```python
from build123d import *

# Parameters (mm, degrees)
BOSS_EXTRUDE1_DEPTH = 25.4
BOSS_EXTRUDE2_DEPTH = 12.7


with BuildPart() as part:
    # Sketch1 → Boss-Extrude1 (new body)
    with BuildSketch(Plane.XY):
        with BuildLine():
            Line((-4.826, 0.016704998), (-4.826, -3.044495583))
            ThreePointArc((-4.826, -3.044495583), (0, -5.698295002), (4.826, -3.044495583))
            Line((4.826, -3.044495583), (4.826, 0.016704998))
            Line((4.826, 0.016704998), (4.826, 3.07790558))
            ThreePointArc((4.826, 3.07790558), (0, 5.731704998), (-4.826, 3.07790558))
            Line((-4.826, 3.07790558), (-4.826, 0.016704998))
        make_face()
    extrude(amount=BOSS_EXTRUDE1_DEPTH)

    # Sketch2 → Boss-Extrude2 (add)
    with BuildSketch(Plane.XY.offset(25.4)):
        with BuildLine():
            Line((0.79375, 0), (0.79375, 1.374815329))
            ThreePointArc((0.79375, 1.374815329), (-1.5875, 0), (0.79375, -1.374815329))
            Line((0.79375, -1.374815329), (0.79375, 0))
        make_face()
    extrude(amount=BOSS_EXTRUDE2_DEPTH)


solid = part.part
```
CAD build for the part. Positions are in the model's coordinates, mm. A direction names the side the tool comes from. Coordinates: 2 decimals unless noted, no trailing zeros. Write each loop counter-clockwise with the first axis right and the second up, starting at its lowest first coordinate (ties: lowest second). Pieces come first, ordered by that corner, then holes.
(1) Cut at D-D, the plane y = 2. List the corners of the cut face in (x, z).
(2) Cut at B-B, the plane y = 0. List the corners of the cut face in (x, z).
(3) Cut at A-A, the plane x = 0. List the corners of the cut face in (y, z).
(4) Flat gauge pins, fed straight in: pin 1 (2 mm diameter, centred on y = 0, z = 30, fed in from +X); pin 2 (1 mm diameter, centred on x = 2, z = 9.5, fed in from -Y); pin 3 (3 mm diameter, centred on x = -2.5, z = 7, fed in from +Y). Where does each tip first touch, or does it go through?
(5) Drill centre lines: probe 1 along Z at (x, y) = (1.5, 2.25); probe 2 along Y at (x, z) = (-0.25, 28); probe 3 along Y at (x, z) = (-1.75, 12.5). Where is each one in solid material? Low to high.
(6) Cut at C-C, the plane z = 20.5. List the corners of the cut face in (x, y) (1 decimal), and give its area (3 significant figures).
(7) 3-axis set-ups, long thin cutter, end or side, ignore diameter. For faces 1 (the face through (-1.587, 0.047, 31.661)), 2 (the face through (0.794, 0, 32)), 3 (the face through (4.826, 0, 13)): which of +Z, -Z, +X, -X, +Y, -Y reach the whole face in a straight line?
Geometry says:
1. outline: (-4.83, 0) - (4.83, 0) - (4.83, 25.4) - (-4.83, 25.4) - close
2. outline: (-4.83, 0) - (4.83, 0) - (4.83, 25.4) - (0.79, 25.4) - (0.79, 38.1) - (-1.59, 38.1) - (-1.59, 25.4) - (-4.83, 25.4) - close
3. outline: (-5.7, 0) - (5.73, 0) - (5.73, 25.4) - (1.59, 25.4) - (1.59, 38.1) - (-1.59, 38.1) - (-1.59, 25.4) - (-5.7, 25.4) - close
4. pin 1: stops at x = 0.79
4. pin 2: stops at y = -5.5
4. pin 3: stops at y = 5.64
5. probe 1: z = 0 to 25.4
5. probe 2: y = -1.57 to 1.57
5. probe 3: y = -5.42 to 5.46
6. outline: (-4.8, -3) arc R5.7 ccw to (4.8, -3) - (4.8, 3.1) arc R5.7 ccw to (-4.8, 3.1) - close
6. area: 95.2 mm2
7. face 1: +Z
7. face 2: +Z, +X, +Y, -Y
7. face 3: +Z, -Z, +X, +Y, -Y
